Can you work these out from the model? Positions are in its coordinate system, mm. Face numbers are marked on the shaded views. A direction names the side the tool comes from. Give positions to 0.01 mm unless a question says otherwise; leave off trailing zeros. Order: outer loops, then holes, each group sorted by start corner. A loop starts at its lowest first (then second) coordinate and runs counter-clockwise, first axis right, second up. Notation, with made-up numbers: (37, 19.25) -> (78, 19.25) arc R15 cw to (78, 42.25) -> close; hole circle Ø11 at (-8.75, 28.5). An arc over 180 degrees is marked (long way). Answer as CSV lines item,"result".
Autodesk Inventor part; units mm, degrees
ref_plane "YZ Plane" through (0, 0, 0) normal (1, 0, 0) x (0, 1, 0)
ref_plane "XZ Plane" through (0, 0, 0) normal (0, 1, 0) x (-1, 0, 0)
ref_plane "XY Plane" through (0, 0, 0) normal (0, 0, 1) x (1, 0, 0)
sketch "Эскиз1" plane through (0, 0, 0) normal (0, 0, 1) x (1, 0, 0)
  line L0 (126.0318, 90) -> (126.0318, -90)
  line L1 (-2.0004, 19) -> (-2.0004, 90)
  circle A0 centre (8.0003, 40) radius 2
  circle A1 centre (8.0003, 0) radius 2
  circle A2 centre (8.0003, -40) radius 2
  circle A3 centre (116.0319, 40) radius 2
  circle A4 centre (116.0319, 0) radius 2
  circle A5 centre (116.0319, -40) radius 2
  line L2 (-2, -79) -> (-2, 19)
  line L3 (-2.0004, -90) -> (-2.0004, -79)
  line L4 (126.0318, 90) -> (-2.0004, 90)
  line L5 (-2.0004, 90) -> (-2.0004, -90)
  line L6 (-2.0004, -90) -> (126.0318, -90)
  line L7 (126.0318, -90) -> (126.0318, 90)
  line L8 (68.0384, 55) -> (18.0384, 55)
  line L9 (18.0384, 55) -> (18.0384, -55)
  line L10 (18.0384, -55) -> (68.0384, -55)
  line L11 (68.0384, -55) -> (68.0384, 55)
  point P0 (0, 0)
  dimension "d0" = 50
  dimension "d1" = 110
  dimension "d2" = 180
  dimension "d3" = 35
extrude "Выдавливание1" add sketch "Эскиз1" along normal blind 3.5
sketch "Эскиз2" plane through (0, 0, 3.5) normal (0, 0, 1) x (1, 0, 0)
  line L0 (18.0384, -55) -> (18.0384, 55)
  line L1 (18.0384, 55) -> (68.0384, 55)
  line L2 (68.0384, 55) -> (68.0384, -55)
  line L3 (68.0384, -55) -> (18.0384, -55)
  line L4 (65.0384, 52) -> (21.0384, 52)
  line L5 (21.0384, 52) -> (21.0384, -52)
  line L6 (21.0384, -52) -> (65.0384, -52)
  line L7 (65.0384, -52) -> (65.0384, 52)
  point P0 (0, 0)
  dimension "d6" = 3
  dimension "d7" = 3
  dimension "d8" = 3
  dimension "d9" = 3
extrude "Выдавливание2" add sketch "Эскиз2" against normal blind 40
sketch "Эскиз3" plane through (0, 0, -36.5) normal (0, 0, -1) x (-1, 0, 0)
  line L0 (-65.0384, -52) -> (-21.0384, -52)
  arc A0 (-34.3523, -52) -> (-51.7245, -52) centre (-43.0384, -55.6937) ccw
  circle A1 centre (-43.0384, -49.8387) radius 2
  line L1 (0, 0) -> (-84.8604, 0) construction
  arc A2 (-51.7245, 52) -> (-34.3523, 52) centre (-43.0384, 55.6937) ccw
  circle A3 centre (-43.0384, 49.8387) radius 2
  line L2 (-34.3523, -52) -> (-51.7245, -52)
  line L3 (-51.7245, 52) -> (-34.3523, 52)
  line L4 (-21.0384, 52) -> (-65.0384, 52)
  dimension "d12" = 44
  dimension "d13" = 22
  dimension "d14" = 4
extrude "Выдавливание3" add sketch "Эскиз3" against normal blind 36.5
sketch "Эскиз4" plane through (21.0384, -52, 3.5) normal (0, 1, 0) x (1, 0, 0)
  line L0 (0, 0) -> (0, 40)
  line L1 (0, 37.0435) -> (9.3788, 37.0435)
  line L2 (9.3788, 37.0435) -> (9.3788, 18.9873)
  line L3 (9.3788, 18.9873) -> (0, 18.9873)
  line L4 (0, 18.9873) -> (0, 37.0435)
  point P0 (-21.0384, 3.5)
extrude "Выдавливание4" cut sketch "Эскиз4" against normal blind 4
equation "\"d3\" = -0.5 * d1 + 0.5 * d2"
properties part number "battery_case"
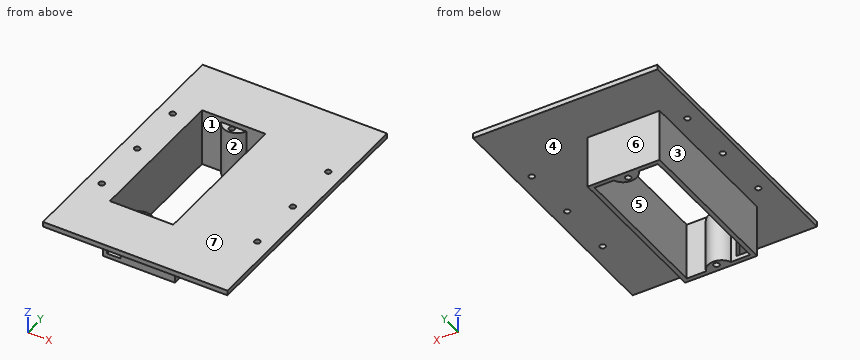
Item 1: For the marked faces 5, 6 and 7, which set-ups out of +Z, -Z, +X, -X, +Y, -Y let a thin tool reach every point of the face, with its end or its side?
Numbers:
face 5,"+Z, -Z"
face 6,"-Z, +X, -X, +Y"
face 7,"+Z, +X, -X, +Y, -Y"
Item 2: Imagine slicing it at A-A, the plane y = 40. Please give me the cut outline in (x, z), then the cut area to 3 significant figures.
Numbers:
outline,"(-2, 0) -> (6, 0) -> (6, 3.5) -> (-2, 3.5) -> close; (10, 0) -> (18.04, 0) -> (18.04, -36.5) -> (21.04, -36.5) -> (21.04, 3.5) -> (10, 3.5) -> close; (65.04, -36.5) -> (68.04, -36.5) -> (68.04, 0) -> (114.03, 0) -> (114.03, 3.5) -> (65.04, 3.5) -> close; (118.03, 0) -> (126.03, 0) -> (126.03, 3.5) -> (118.03, 3.5) -> close"
area,"485 mm²"
Item 3: We'd pull the mould along X, two halves only. Please class the marked faces 1, 2, 3 and 4: released by +X, released by -X, zero draft, split by the parting line, or undercut.
Numbers:
face 1,"undercut"
face 2,"undercut"
face 3,"released by -X"
face 4,"zero draft"
Item 4: Please list where these lines run through material, in increasing order: line 1 along Y through (x, z) = (43, -12); line 2 along Y through (x, z) = (23, -13); line 3 along X through (y, z) = (-8.5, -7.5).
Numbers:
line 1,"y = -55 to -51.84, -47.84 to -46.25, 46.25 to 47.84, 51.84 to 55"
line 2,"y = -55 to -52, 52 to 55"
line 3,"x = 18.04 to 21.04, 65.04 to 68.04"
Item 5: Imagine slicing it at C-C, the plane y = -35. Please give me the cut outline in (x, z), then the cut area to 3 significant figures.
Numbers:
outline,"(-2, 0) -> (18.04, 0) -> (18.04, -36.5) -> (21.04, -36.5) -> (21.04, 3.5) -> (-2, 3.5) -> close; (65.04, -36.5) -> (68.04, -36.5) -> (68.04, 0) -> (126.03, 0) -> (126.03, 3.5) -> (65.04, 3.5) -> close"
area,"513 mm²"
Item 6: Imagine slicing it at D-D, the plane y = 59.5. Please give me the cut outline in (x, z).
Numbers:
outline,"(-2, 0) -> (126.03, 0) -> (126.03, 3.5) -> (-2, 3.5) -> close"
Item 7: Imagine slicing it at B-B, the plane z = -24.5. Please give me the cut outline in (x, y), then the cut area to 3 significant figures.
Numbers:
outline,"(18.04, -55) -> (21.04, -55) -> (21.04, 52) -> (34.35, 52) arc R9.44 ccw to (51.72, 52) -> (65.04, 52) -> (65.04, -52) -> (51.72, -52) arc R9.44 ccw to (34.35, -52) -> (30.42, -52) -> (30.42, -55) -> (68.04, -55) -> (68.04, 55) -> (18.04, 55) -> close; hole circle Ø4 at (43.04, -49.84); hole circle Ø4 at (43.04, 49.84)"
area,"1,010 mm²"
Item 8: For pin 1 (11 mm diameter, centred on x = 42, z = -17, fed in from +Y); pin 2 (8 mm diameter, centred on y = -52.5, z = -9, fed in from +X); pin 3 (2.5 mm diameter, centred on y = -53.5, z = -25, fed in from -X), each with a flat end and sliding along its axis, tell me the tip position at first contact or that it passes through.
Numbers:
pin 1,"stops at y = 55"
pin 2,"stops at x = 68.04"
pin 3,"stops at x = 18.04"
